Part model, mm, in its own coordinate system. Round coordinates to 2 decimals unless told otherwise and drop trailing zeros. Order: outer loops, then holes, each group sorted by start corner. A loop starts at its lowest first (then second) coordinate and runs counter-clockwise, first axis right, second up. Notation, with made-up numbers: (66.5, 7.5) -> (71.5, 7.5) arc R11 ccw to (71.5, 15.5) -> close; hole circle Ø6 at (81.5, -1.5). An arc over 180 degrees is marked (long way). Use CSV: the item, a comma, the result in double quotes.
Autodesk Inventor part; units mm, degrees
ref_plane "YZ Plane" through (0, 0, 0) normal (1, 0, 0) x (0, 1, 0)
ref_plane "XZ Plane" through (0, 0, 0) normal (0, 1, 0) x (-1, 0, 0)
ref_plane "XY Plane" through (0, 0, 0) normal (0, 0, 1) x (1, 0, 0)
sketch "Sketch1" plane through (0, 0, 0) normal (1, 0, 0) x (0, 1, 0)
  line L0 (45.75, 25) -> (-45.75, 25)
  line L1 (-45.75, 25) -> (-45.75, -25)
  line L2 (-45.75, -25) -> (45.75, -25)
  line L3 (45.75, -25) -> (45.75, 25)
  circle A0 centre (44, 22) radius 1.25
  line L4 (0, 25) -> (0, -25) construction
  circle A1 centre (-44, 22) radius 1.25
  line L5 (-34, 25) -> (-34, 31)
  line L6 (-34, 31) -> (34, 31)
  line L7 (34, 31) -> (34, 25)
  line L8 (-31.75, -12) -> (-20.75, -12)
  line L9 (-20.75, -12) -> (-20.75, -13)
  line L10 (-20.75, -13) -> (-31.75, -13)
  line L11 (-31.75, -13) -> (-31.75, -12)
  line L12 (31.75, -12) -> (20.75, -12)
  line L13 (20.75, -12) -> (20.75, -13)
  line L14 (20.75, -13) -> (31.75, -13)
  line L15 (31.75, -13) -> (31.75, -12)
  line L16 (-39.75, 7) -> (-40.75, 7)
  line L17 (-40.75, 7) -> (-40.75, -4)
  line L18 (-40.75, -4) -> (-39.75, -4)
  line L19 (-39.75, -4) -> (-39.75, 7)
  line L20 (39.75, 7) -> (40.75, 7)
  line L21 (40.75, 7) -> (40.75, -4)
  line L22 (40.75, -4) -> (39.75, -4)
  line L23 (39.75, -4) -> (39.75, 7)
  circle A2 centre (0, -5) radius 1.25
  circle A3 centre (0, 54.3) radius 1.25
  line L24 (22, 31) -> (22, 37)
  line L25 (22, 37) -> (9, 37)
  line L26 (9, 37) -> (9, 57.5)
  line L27 (-9, 57.5) -> (-9, 37)
  line L28 (-9, 37) -> (-22, 37)
  line L29 (-22, 37) -> (-22, 31)
  line L30 (9, 57.5) -> (-9, 57.5)
  circle A4 centre (0, 32.7) radius 1.25
  point P0 (0, 0)
  point P1 (45.75, 0)
  dimension "d0" = 50
  dimension "d1" = 91.5
  dimension "d2" = 2.5
  dimension "d4" = 3
  dimension "d11" = 11.75
  dimension "d12" = 6
  dimension "d13" = 11.75
  dimension "d18" = 1
  dimension "d19" = 11
  dimension "d20" = 14
  dimension "d21" = 12
  dimension "d24" = 21
  dimension "d25" = 1
  dimension "d26" = 5
  dimension "d27" = 11
  dimension "d28" = 30
  dimension "d29" = 2.5
  dimension "d30" = 2.5
  dimension "d33" = 6
  dimension "d34" = 25
  dimension "d35" = 25
  dimension "d37" = 12
  dimension "d38" = 12
  dimension "d39" = 9
  dimension "d41" = 26.5
  dimension "d42" = 3.2
  dimension "d43" = 2.5
  dimension "d44" = 37.7
  dimension "d45" = 10
extrude "Extrusion1" add sketch "Sketch1" along normal blind 1 contours L3 L2 L1 L0 | L0 L5 L6 L7 | L6 L29 L28 L27 L30 L26 L25 L24 | L8 L9 L10 L11 | L15 L14 L13 L12 | L19 L18 L17 L16 | L20 L21 L22 L23 | A2 | A3 | A4
fillet "Fillet1" radius 2 10 edges at (0.5, -45.75, 25) (0.5, -34, 31) (0.5, 34, 31) (0.5, 45.75, 25) (0.5, -45.75, -25) (0.5, 45.75, -25) (0.5, 9, 57.5) (0.5, -9, 57.5) (0.5, 22, 37) (0.5, -22, 37)
extrude "Extrusion2" cut sketch "Sketch1" along normal up to next contours L8 L9 L10 L11 | L15 L14 L13 L12 | L19 L18 L17 L16 | L20 L21 L22 L23 | A2 | A3 | A4
properties part number "PCB"
(1) Cut at D-D, the plane y = -19. Give the cut face in (x, z).
Reply:
outline,"(0, -25) -> (1, -25) -> (1, 37) -> (0, 37) -> close"
(2) Cut at C-C, the plane x = 0.3. State how many separate pieces and enclosed holes the cut face has, then the cut area to 3 significant figures.
Reply:
separate pieces,"1"
enclosed holes,"9"
area,"5,540 mm2"
(3) Pull direction Z, two halves, no side cores. Call faces 1 (the face through (0.49, -0.27, 55.52)), 2 (the face through (0.51, -45.15, 24.43)), 3 (the face through (0.51, 45.15, -24.43)): released by +Z, released by -Z, zero draft, split by the parting line, or undercut.
Reply:
face 1,"undercut"
face 2,"released by +Z"
face 3,"released by -Z"
(4) Cut at B-B, the plane z = 54.3. Give the cut face in (x, y).
Reply:
outline,"(0, -9) -> (1, -9) -> (1, -1.25) -> (0, -1.25) -> close; (0, 1.25) -> (1, 1.25) -> (1, 9) -> (0, 9) -> close"
(5) Drop flat-ended pins along their axis: P1, Ø0.5, axis at x = 0.5, z = 27.5, coming from the -Y side; P2, Ø2, axis at y = -44, z = 22, coming from the +X side. Give the stop position or say it passes through.
Reply:
P1,"y = -34"
P2,"through"
(6) Cut at A-A, the plane z = 22. Give the cut face in (x, y).
Reply:
outline,"(0, -45.75) -> (1, -45.75) -> (1, -45.25) -> (0, -45.25) -> close; (0, -42.75) -> (1, -42.75) -> (1, 42.75) -> (0, 42.75) -> close; (0, 45.25) -> (1, 45.25) -> (1, 45.75) -> (0, 45.75) -> close"
(7) Probe probe 1 along Z at (x, y) = (0.6, 0); probe 2 along Y at (x, z) = (0.5, 5); probe 3 along Z at (x, y) = (0.4, -24). List the from-to ranges inside material, lowest first. Write a range as [from, to].
Reply:
probe 1,"[-25, -6.25], [-3.75, 31.45], [33.95, 53.05], [55.55, 57.5]"
probe 2,"[-45.75, -40.75], [-39.75, 39.75], [40.75, 45.75]"
probe 3,"[-25, -13], [-12, 31]"
